Here's how the part is built. I have some questions about the finished solid (model axes, mm). Face numbers are marked on the shaded views. A direction names the side the tool comes from. Round coordinates to 2 decimals unless told otherwise and drop trailing zeros. Order: outer loops, then holes, each group sorted by start corner. A loop starts at its lowest first (then second) coordinate and runs counter-clockwise, first axis right, second up. Notation, with made-up numbers: (37.25, -1) -> (87.25, -1) arc R31 cw to (87.25, 29) -> close; hole circle Ø7 at (25.5, 37.5). An arc over 180 degrees is marked (long way). Answer in a Markdown table with one row per item.
```python
from build123d import *

# Parameters (mm, degrees)
SKETCH1_W           = 64.757022316
SKETCH1_H           = 64.860932096
SKETCH1_R           = 0.635
BOSS_EXTRUDE1_DEPTH = 5.08
SKETCH2_R           = 19.05
BOSS_EXTRUDE2_DEPTH = 5.08
SKETCH3_R           = 3.175
BOSS_EXTRUDE3_DEPTH = 2.54


with BuildPart() as part:
    # Sketch1 → Boss-Extrude1 (new body)
    with BuildSketch(Plane(origin=(0, 0, 0), x_dir=(1, 0, 0), z_dir=(0, 1, 0))):
        Rectangle(SKETCH1_W, SKETCH1_H)
        with Locations(Location((-28.575, 28.575, 0), (0, 0, 270))):
            Circle(SKETCH1_R, mode=Mode.SUBTRACT)
        with Locations(Location((-23.495, 28.575, 0), (0, 0, 270))):
            Circle(SKETCH1_R, mode=Mode.SUBTRACT)
        with Locations(Location((-28.575, 23.495, 0), (0, 0, 270))):
            Circle(SKETCH1_R, mode=Mode.SUBTRACT)
        with Locations(Location((28.575, 28.575, 0), (0, 0, 270))):
            Circle(SKETCH1_R, mode=Mode.SUBTRACT)
        with Locations(Location((23.495, 28.575, 0), (0, 0, 270))):
            Circle(SKETCH1_R, mode=Mode.SUBTRACT)
        with Locations(Location((28.575, 23.495, 0), (0, 0, 270))):
            Circle(SKETCH1_R, mode=Mode.SUBTRACT)
        with Locations(Location((28.575, -28.575, 0), (0, 0, 270))):
            Circle(SKETCH1_R, mode=Mode.SUBTRACT)
        with Locations(Location((28.575, -23.495, 0), (0, 0, 270))):
            Circle(SKETCH1_R, mode=Mode.SUBTRACT)
        with Locations(Location((23.495, -28.575, 0), (0, 0, 270))):
            Circle(SKETCH1_R, mode=Mode.SUBTRACT)
        with Locations(Location((-28.575, -28.575, 0), (0, 0, 270))):
            Circle(SKETCH1_R, mode=Mode.SUBTRACT)
        with Locations(Location((-28.575, -23.495, 0), (0, 0, 270))):
            Circle(SKETCH1_R, mode=Mode.SUBTRACT)
        with Locations(Location((-23.495, -28.575, 0), (0, 0, 270))):
            Circle(SKETCH1_R, mode=Mode.SUBTRACT)
    extrude(amount=BOSS_EXTRUDE1_DEPTH)

    # Sketch2 → Boss-Extrude2 (add)
    with BuildSketch(Plane(origin=(0, 5.08, 0), x_dir=(1, 0, 0), z_dir=(0, 1, 0))):
        with Locations(Location((0, 0, 0), (0, 0, 270))):
            Circle(SKETCH2_R)
    extrude(amount=BOSS_EXTRUDE2_DEPTH)

    # Sketch3 → Boss-Extrude3 (add)
    with BuildSketch(Plane(origin=(0, 10.16, 0), x_dir=(1, 0, 0), z_dir=(0, 1, 0))):
        with Locations(Location((0, 0, 0), (0, 0, 270))):
            Circle(SKETCH3_R)
    extrude(amount=BOSS_EXTRUDE3_DEPTH)


solid = part.part
```
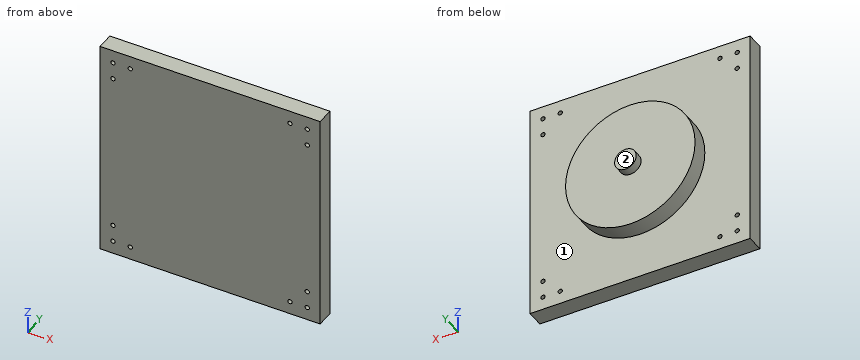
1. Please list where these lines run through material, in increasing order: line 1 along Z through (x, y) = (29, 3); line 2 along X through (y, z) = (1.75, 28.5); line 3 along X through (y, z) = (1.75, -29).
Numbers:
| item | result |
|---|---|
| line 1 | z = -32.43 to -29.05, -28.1 to -23.97, -23.02 to 23.02, 23.97 to 28.1, 29.05 to 32.43 |
| line 2 | x = -32.38 to -29.21, -27.94 to -24.13, -22.86 to 22.86, 24.13 to 27.94, 29.21 to 32.38 |
| line 3 | x = -32.38 to -29.05, -28.1 to -23.97, -23.02 to 23.02, 23.97 to 28.1, 29.05 to 32.38 |
2. For the marked faces 1 and 2, which set-ups out of +Z, -Z, +X, -X, +Y, -Y let a thin tool reach every point of the face, with its end or its side?
Numbers:
| item | result |
|---|---|
| face 1 | +Y |
| face 2 | +Z, -Z, +X, -X, +Y |
3. Suppose I cut it at A-A on z = 0. Write out the boundary of the cut face in (x, y) (3 decimals).
Numbers:
| item | result |
|---|---|
| outline | (-32.379, 0) -> (32.379, 0) -> (32.379, 5.08) -> (19.05, 5.08) -> (19.05, 10.16) -> (3.175, 10.16) -> (3.175, 12.7) -> (-3.175, 12.7) -> (-3.175, 10.16) -> (-19.05, 10.16) -> (-19.05, 5.08) -> (-32.379, 5.08) -> close |
4. Suppose I cut it at B-B on x = 0. Write out the boundary of the cut face in (y, z) (3 decimals).
Numbers:
| item | result |
|---|---|
| outline | (0, -32.43) -> (5.08, -32.43) -> (5.08, -19.05) -> (10.16, -19.05) -> (10.16, -3.175) -> (12.7, -3.175) -> (12.7, 3.175) -> (10.16, 3.175) -> (10.16, 19.05) -> (5.08, 19.05) -> (5.08, 32.43) -> (0, 32.43) -> close |
5. Suppose I cut it at C-C on y = 9. Write out the boundary of the cut face in (x, z), then the cut area to 3 significant figures.
Numbers:
| item | result |
|---|---|
| outline | circle Ø38.1 at (0, 0) |
| area | 1,140 mm2 |
6. For pin 1 Ø1.1 at (x, z) = (-28.575, 23.495) entering from +Y; pin 2 Ø4 at (x, y) = (14.5, 8) entering from +Z; pin 3 Ø10 at (x, z) = (9.5, -21) entering from +Y; pin 4 Ø2 at (x, z) = (23.495, 28.575) entering from +Y, each with a flat end and sliding along its axis, tell me the tip position at first contact or that it passes through.
Numbers:
| item | result |
|---|---|
| pin 1 | passes through |
| pin 2 | stops at z = 14.38 |
| pin 3 | stops at y = 10.16 |
| pin 4 | stops at y = 5.08 |
7. Suppose I cut it at D-D on x = -17.5. Write out the boundary of the cut face in (y, z), then the cut area to 3 significant figures.
Numbers:
| item | result |
|---|---|
| outline | (0, -32.43) -> (5.08, -32.43) -> (5.08, -7.53) -> (10.16, -7.53) -> (10.16, 7.53) -> (5.08, 7.53) -> (5.08, 32.43) -> (0, 32.43) -> close |
| area | 406 mm2 |
